Could you check a few things on this model? Use its own coordinates, in mm. Coordinates: 2 decimals unless noted, no trailing zeros. Loops run counter-clockwise (first coordinate to the right, second up) from the corner with the lowest first, then second, coordinate; pieces in that order, holes last. Notation, with made-up numbers: M -5.5,-10.75 L 1.5,-10.75 A31 ccw 1.5,19.25 Z; hole C 52,37.5 d9. An arc over 180 degrees is marked long. Write each question's results on one line, items separated by ' | '.
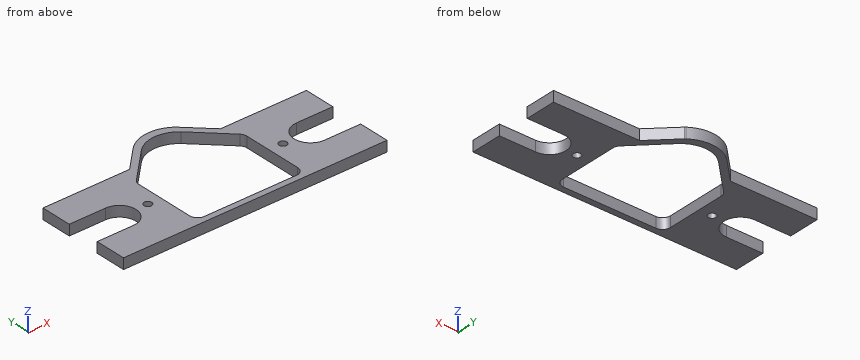
Autodesk Inventor part; units mm, degrees
ref_plane "YZ Plane" through (0, 0, 0) normal (1, 0, 0) x (0, 1, 0)
ref_plane "XZ Plane" through (0, 0, 0) normal (0, 1, 0) x (-1, 0, 0)
ref_plane "XY Plane" through (0, 0, 0) normal (0, 0, 1) x (1, 0, 0)
sketch "Block1" plane through (0, 0, 0) normal (0, 0, 1) x (1, 0, 0)
  line L0 (-17.5911, -8.406) -> (-17.5911, -2.6569)
  arc A0 (-15.6308, 0.6431) -> (-17.4939, -2.2845) centre (9.5285, -17.4245) ccw
  arc A1 (-17.4939, -2.2845) -> (-17.5911, -2.6569) centre (-16.8291, -2.6569) ccw
  line L1 (-13.0521, -3.6322) -> (-2.9855, -3.6322)
  line L2 (-2.9855, -3.6322) -> (-2.9855, -10.0136)
  line L3 (-2.9855, -10.0136) -> (-13.0521, -10.0136)
  line L4 (-13.0521, -10.0136) -> (-13.0521, -3.6322)
  ellipse E0 centre (-8.0188, -3.6322) end of major axis (-8.0188, -7.4704) minor radius 2.9685
  point P0 (-13.9703, -5.5207)
  point P1 (-17.5911, -2.4593)
  dimension "d111" = 0.762
sketch "Block2" plane through (0, 0, 0) normal (0, 0, 1) x (1, 0, 0)
  line L0 (-7.8958, -2.4967) -> (-7.8958, -8.4058)
  line L1 (-8.6339, -9.168) -> (-16.8291, -9.168)
  ellipse E0 centre (-12.6564, -2.1178) end of major axis (-12.6564, -6.4967) minor radius 3.853 (-9.6585, 0.6329) -> (-15.6415, 0.6509) ccw
  arc A0 (-7.8958, -2.4967) -> (-9.6091, 0.6391) centre (-35.8892, -15.7554) ccw
  line L2 (-17.6018, -8.3981) -> (-17.6018, -2.6491)
  arc A1 (-15.6415, 0.6509) -> (-17.5045, -2.2766) centre (9.5178, -17.4167) ccw
  arc A2 (-17.5045, -2.2766) -> (-17.6018, -2.6491) centre (-16.8398, -2.6491) ccw
  line L3 (-13.0627, -3.6243) -> (-2.9962, -3.6243)
  line L4 (-2.9962, -3.6243) -> (-2.9962, -10.0058)
  line L5 (-2.9962, -10.0058) -> (-13.0627, -10.0058)
  line L6 (-13.0627, -10.0058) -> (-13.0627, -3.6243)
  ellipse E1 centre (-8.0295, -3.6243) end of major axis (-8.0295, -7.4625) minor radius 2.9685
  point P0 (-12.2397, -5.1213)
sketch "Block3" plane through (0, 0, 0) normal (0, 0, 1) x (1, 0, 0)
  arc A0 (-17.5911, -8.406) -> (-16.8291, -9.168) centre (-16.8291, -8.406) ccw
  arc A1 (-8.6339, -9.168) -> (-7.8719, -8.406) centre (-8.6339, -8.406) ccw
  line L0 (-7.8958, -2.4967) -> (-7.8958, -8.4058)
  line L1 (-8.6339, -9.168) -> (-16.8291, -9.168)
  ellipse E0 centre (-12.6564, -2.1178) end of major axis (-12.6564, -6.4967) minor radius 3.853 (-9.6585, 0.6329) -> (-15.6415, 0.6509) ccw
  arc A2 (-7.8958, -2.4967) -> (-9.6091, 0.6391) centre (-35.8892, -15.7554) ccw
  line L2 (-17.6018, -8.3981) -> (-17.6018, -2.6491)
  arc A3 (-15.6415, 0.6509) -> (-17.5045, -2.2766) centre (9.5178, -17.4167) ccw
  arc A4 (-17.5045, -2.2766) -> (-17.6018, -2.6491) centre (-16.8398, -2.6491) ccw
  line L3 (-13.0627, -3.6243) -> (-2.9962, -3.6243)
  line L4 (-2.9962, -3.6243) -> (-2.9962, -10.0058)
  line L5 (-2.9962, -10.0058) -> (-13.0627, -10.0058)
  line L6 (-13.0627, -10.0058) -> (-13.0627, -3.6243)
  ellipse E1 centre (-8.0295, -3.6243) end of major axis (-8.0295, -7.4625) minor radius 2.9685
  point P0 (-12.6868, -8.3844)
  dimension "d110" = 0.762
sketch "Block4" plane through (0, 0, 0) normal (0, 0, 1) x (1, 0, 0)
  arc A0 (-17.5911, -8.406) -> (-16.8291, -9.168) centre (-16.8291, -8.406) ccw
  arc A1 (-8.6339, -9.168) -> (-7.8719, -8.406) centre (-8.6339, -8.406) ccw
  line L0 (-7.8958, -2.4967) -> (-7.8958, -8.4058)
  line L1 (-8.6339, -9.168) -> (-16.8291, -9.168)
  ellipse E0 centre (-12.6564, -2.1178) end of major axis (-12.6564, -6.4967) minor radius 3.853 (-9.6585, 0.6329) -> (-15.6415, 0.6509) ccw
  arc A2 (-7.8958, -2.4967) -> (-9.6091, 0.6391) centre (-35.8892, -15.7554) ccw
  line L2 (-17.6018, -8.3981) -> (-17.6018, -2.6491)
  arc A3 (-15.6415, 0.6509) -> (-17.5045, -2.2766) centre (9.5178, -17.4167) ccw
  arc A4 (-17.5045, -2.2766) -> (-17.6018, -2.6491) centre (-16.8398, -2.6491) ccw
  line L3 (-13.0627, -3.6243) -> (-2.9962, -3.6243)
  line L4 (-2.9962, -3.6243) -> (-2.9962, -10.0058)
  line L5 (-2.9962, -10.0058) -> (-13.0627, -10.0058)
  line L6 (-13.0627, -10.0058) -> (-13.0627, -3.6243)
  ellipse E1 centre (-8.0295, -3.6243) end of major axis (-8.0295, -7.4625) minor radius 2.9685
  point P0 (-12.6868, -8.3844)
sketch "Block5" plane through (0, 0, 0) normal (0, 0, 1) x (1, 0, 0)
  ellipse E0 centre (-12.7876, -1.8459) end of major axis (-12.7876, -5.6516) minor radius 3.3457 (-10.6846, 1.114) -> (-14.8941, 1.1109) ccw
  arc A0 (-15.6984, 0.3796) -> (-14.8859, 1.1184) centre (-85.8065, 78.298) ccw
  arc A1 (-10.6894, 1.1184) -> (-9.8669, 0.3716) centre (60.1779, 78.3469) ccw
  point P0 (-12.7899, 8.9309)
sketch "Block6" plane through (0, 0, 0) normal (0, 0, 1) x (1, 0, 0)
  arc A0 (-10.9697, 1.4333) -> (-15.1792, 1.1122) centre (-12.8849, -1.2117) ccw
  line L0 (-15.1792, 1.1122) -> (-17.7718, -1.4473)
  line L1 (-10.8839, 1.361) -> (-8.0119, -1.4473)
  line L2 (-17.7718, -1.4473) -> (-8.0119, -1.4473)
  arc A1 (-10.8839, 1.361) -> (-10.9697, 1.4333) centre (-11.4166, 0.8161) ccw
  point P0 (-12.0633, -0.3449)
  point P1 (-10.9214, 1.3977)
  dimension "d153" = 0.762
sketch "Sketch1" plane through (0, 0, 0) normal (0, 0, 1) x (1, 0, 0)
  line L0 (-25.4704, -0.3682) -> (-0.0704, -0.3682)
  line L1 (-0.0704, -0.3682) -> (-0.0704, -9.5122)
  line L2 (-0.0704, -9.5122) -> (-25.4704, -9.5122)
  line L3 (-25.4704, -9.5122) -> (-25.4704, -0.3682)
extrude "Extrusion1" add sketch "Sketch1" along normal blind 1.016
sketch "Sketch2" plane through (0, 0, 1.016) normal (0, 0, 1) x (1, 0, 0)
  line L0 (-15.6279, -1.8922) -> (-9.9129, -1.8922)
  line L1 (-8.3254, -3.4797) -> (-8.3254, -6.4007)
  line L2 (-9.9129, -7.9882) -> (-15.6279, -7.9882)
  line L3 (-17.2154, -6.4007) -> (-17.2154, -3.4797)
  arc A0 (-15.6279, -1.8922) -> (-17.2154, -3.4797) centre (-15.6279, -3.4797) ccw
  arc A1 (-17.2154, -6.4007) -> (-15.6279, -7.9882) centre (-15.6279, -6.4007) ccw
  arc A2 (-9.9129, -7.9882) -> (-8.3254, -6.4007) centre (-9.9129, -6.4007) ccw
  arc A3 (-8.3254, -3.4797) -> (-9.9129, -1.8922) centre (-9.9129, -3.4797) ccw
extrude "Extrusion2" cut sketch "Sketch2" against normal blind 1.016
sketch "Sketch3" plane through (0, 0, 1.016) normal (0, 0, 1) x (1, 0, 0)
  line L0 (-0.0704, -0.3682) -> (-0.0704, -9.5122)
  line L1 (-25.4704, -9.5122) -> (-25.4704, -0.3682)
  line L2 (-0.0704, -9.5122) -> (-25.4704, -9.5122)
  line L3 (-25.4704, -3.3527) -> (-21.9779, -3.3527)
  line L4 (-20.3904, -4.9402) -> (-20.3904, -4.9402)
  line L5 (-21.9779, -6.5277) -> (-25.4704, -6.5277)
  arc A0 (-20.3904, -4.9402) -> (-21.9779, -3.3527) centre (-21.9779, -4.9402) ccw
  arc A1 (-21.9779, -6.5277) -> (-20.3904, -4.9402) centre (-21.9779, -4.9402) ccw
  line L6 (-0.0704, -3.3527) -> (-3.5629, -3.3527)
  line L7 (-5.1504, -4.9402) -> (-5.1504, -4.9402)
  line L8 (-3.5629, -6.5277) -> (-0.0704, -6.5277)
  arc A2 (-3.5629, -3.3527) -> (-5.1504, -4.9402) centre (-3.5629, -4.9402) ccw
  arc A3 (-5.1504, -4.9402) -> (-3.5629, -6.5277) centre (-3.5629, -4.9402) ccw
extrude "Extrusion3" cut sketch "Sketch3" against normal blind 1.016
sketch "Sketch13" plane through (0, 0, 1.016) normal (0, 0, 1) x (1, 0, 0)
  arc A0 (-10.8192, 2.023) -> (-15.0287, 1.7019) centre (-12.7344, -0.622) ccw
  line L0 (-15.0287, 1.7019) -> (-17.6213, -0.8576)
  line L1 (-10.7334, 1.9507) -> (-7.8614, -0.8576)
  line L2 (-17.6213, -0.8576) -> (-7.8614, -0.8576)
  arc A1 (-10.7334, 1.9507) -> (-10.8192, 2.023) centre (-11.2661, 1.4058) ccw
  point P0 (0, 0)
  point P1 (0, 0)
  point P2 (0, 0)
extrude "Extrusion8" add sketch "Sketch13" against normal blind 1.016
sketch "Sketch12" plane through (0, 0, 1.016) normal (0, 0, 1) x (1, 0, 0)
  line L0 (-7.5424, -2.4012) -> (-7.5424, -8.1771)
  line L1 (-8.3044, -8.9391) -> (-17.2004, -8.9391)
  line L2 (-17.9624, -2.4) -> (-17.9624, -8.1771)
  arc A0 (-17.9624, -8.1771) -> (-17.2004, -8.9391) centre (-17.2004, -8.1771) ccw
  arc A1 (-8.3044, -8.9391) -> (-7.5424, -8.1771) centre (-8.3044, -8.1771) ccw
  line L3 (-10.8562, 1.2031) -> (-7.7678, -1.8602)
  line L4 (-14.7403, 1.0994) -> (-17.7357, -1.8577)
  arc A2 (-10.847, 1.1949) -> (-14.7403, 1.0994) centre (-12.7429, -0.9239) ccw
  arc A3 (-17.7357, -1.8577) -> (-17.9624, -2.4) centre (-17.2004, -2.4) ccw
  arc A4 (-7.5424, -2.4012) -> (-7.7678, -1.8602) centre (-8.3044, -2.4012) ccw
  point P0 (0, 0)
  point P1 (-17.1532, -8.9391)
  point P2 (-17.9624, -7.9131)
  point P3 (-7.5424, -8.1803)
  point P4 (-8.3956, -8.9391)
  point P5 (0, 0)
  point P6 (-17.6124, -1.736)
  point P7 (-17.9624, -2.2782)
  point P8 (-7.8931, -1.7359)
  point P9 (-7.5424, -2.2782)
  dimension "d149" = 0.762
  dimension "d150" = 0.762
  dimension "d154" = 0.762
extrude "Extrusion7" cut sketch "Sketch12" against normal blind 1.016
hole "Hole9" at (-19.2355, -4.93, 1.016) direction (0, 0, -1) diameter 0.7366 depth 1.524
hole "Hole10" at (-6.1975, -4.9172, 1.016) direction (0, 0, -1) diameter 0.7366 depth 2.794
properties part number "headplateLP_tapped"
(1) Please list where these lines run through material, in increasing order: probe 1 along X at (y, z) = (-4.93, 0.35); probe 2 along Y at (x, z) = (-1.75, 0.2); probe 3 along X at (y, z) = (-6.75, 0.45). Write a range as from..to.
Reported:
probe 1: x = -20.39..-19.6, -18.87..-17.96, -7.54..-6.57, -5.83..-5.15 | probe 2: y = -9.51..-6.53, -3.35..-0.37 | probe 3: x = -25.47..-17.96, -7.54..-0.07
(2) Imagine slicing it at D-D, the plane y = -4.93. List the corners of the cut face in (x, z) for me.
Reported:
outline: M -20.39,0 L -19.6,0 L -19.6,1.02 L -20.39,1.02 Z; M -18.87,0 L -17.96,0 L -17.96,1.02 L -18.87,1.02 Z; M -7.54,0 L -6.57,0 L -6.57,1.02 L -7.54,1.02 Z; M -5.83,0 L -5.15,0 L -5.15,1.02 L -5.83,1.02 Z
(3) Imagine slicing it at A-A, the plane y = -8.5. List the corners of the cut face in (x, z) for me, and give its area (3 significant figures).
Reported:
outline: M -25.47,0 L -17.89,0 L -17.89,1.02 L -25.47,1.02 Z; M -7.61,0 L -0.07,0 L -0.07,1.02 L -7.61,1.02 Z | area: 15.4 mm2
(4) Imagine slicing it at B-B, the plane x = -21. List the corners of the cut face in (y, z) for me.
Reported:
outline: M -9.51,0 L -6.19,0 L -6.19,1.02 L -9.51,1.02 Z; M -3.69,0 L -0.37,0 L -0.37,1.02 L -3.69,1.02 Z
(5) Imagine slicing it at C-C, the plane z = 0.3. State how many separate pieces and enclosed holes the cut face has, and give its area (3 significant figures).
Reported:
separate pieces: 1 | enclosed holes: 3 | area: 122 mm2
(6) Will these pins go through, and if not, where does the flat tip stop? P1, Ø0.5, axis at y = -4.5, z = 0.5, coming from the +X side; P2, Ø0.5, axis at x = -12.5, z = 0.5, coming from the +Y side.
Reported:
P1: stops at x = -4.99 | P2: stops at y = 2.64
